Answer from the drawing. Dimensions are ordinates in mm from the lowest x, y and z of the part. Give positions to 0.01 mm unless a question says otherwise; leave off trailing zeros. Loops run counter-clockwise (first coordinate to the right, second up) from the corner with the lowest first, then second, coordinate; pieces in that order, holes last. Notation, with made-up numbers: (-17.5, 61) - (20.5, 61) arc R19 cw to (20.5, 81) - close; hole circle Ø6 at (61, 26). An arc over 180 degrees is marked (long way). Put each result on its own line as item: value. Start each with the question number.
1. A cutting plane is placed at D-D, the plane z = 47. Determine the outline of the cut face in (x, y), plus the area to 3 significant figures.
2. Consider L1, parallel to X at y = 6.5, z = 27.5; L2, parallel to Z at x = 25, y = 2.25 (1 decimal); L3, parallel to X at y = 6.75, z = 44.5 (1 decimal). Determine where each line is inside the solid, lowest interval first. Write a range as from..to.
3. A cutting plane is placed at C-C, the plane y = 2.75. Determine the outline of the cut face in (x, z) (1 decimal).
4. For a pull along Z with two mould halves and no side action, classify the marked faces 1, 2 and 3 as released by +Z, released by -Z, zero draft, split by the parting line, or undercut.
5. A cutting plane is placed at B-B, the plane x = 27.5. Determine the outline of the cut face in (y, z), plus the area to 3 significant figures.
6. Given pin 1 Ø1.5 at (y, z) = (3.5, 24) entering from -X; pin 2 Ø2 at (y, z) = (3.5, 20) entering from -X; pin 3 Ø1.2 at (x, z) = (34, 18) entering from +Y; pin 4 Ø13.5 at (x, z) = (27.5, 27.5) entering from -Y, each flat-ended and moving along its own axis, determine where each tip first touches the part or whether it passes through.
7. A cutting plane is placed at A-A, the plane z = 27.5. Determine the outline of the cut face in (x, y), plus the area to 3 significant figures.
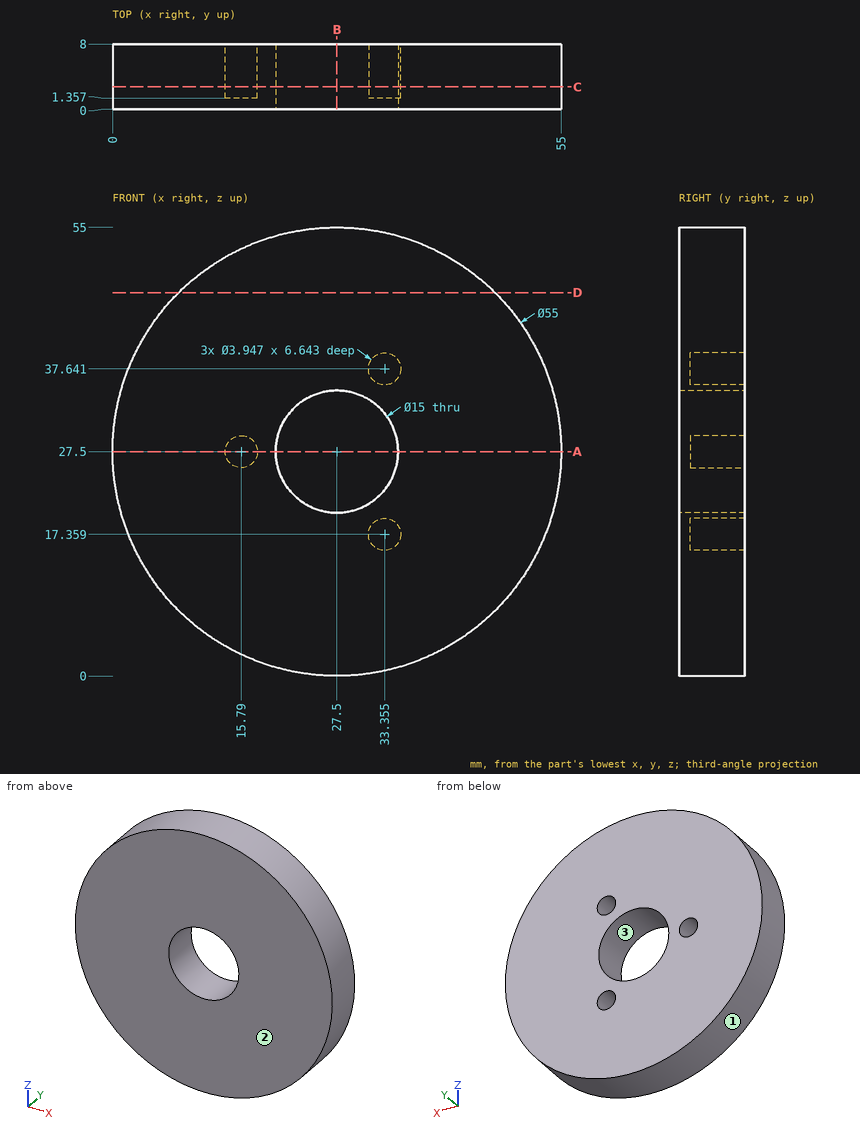
Return value:
1. outline: (8.11, 0) - (46.89, 0) - (46.89, 8) - (8.11, 8) - close
1. area: 310 mm2
2. L1: x = 0..13.82, 17.76..20, 35..55
2. L2: z = 0.1..20.4, 34.6..54.9
2. L3: x = 5.9..49.1
3. outline: circle Ø55 at (27.5, 27.5); hole circle Ø3.9 at (15.8, 27.5); hole circle Ø15 at (27.5, 27.5); hole circle Ø3.9 at (33.4, 17.4); hole circle Ø3.9 at (33.4, 37.6)
4. face 1: split by the parting line
4. face 2: zero draft
4. face 3: undercut
5. outline: (0, 0) - (8, 0) - (8, 20) - (0, 20) - close; (0, 35) - (8, 35) - (8, 55) - (0, 55) - close
5. area: 320 mm2
6. pin 1: stops at x = 0.14
6. pin 2: stops at x = 0.78
6. pin 3: stops at y = 1.36
6. pin 4: passes through
7. outline: (0, 0) - (20, 0) - (20, 8) - (17.76, 8) - (17.76, 1.36) - (13.82, 1.36) - (13.82, 8) - (0, 8) - close; (35, 0) - (55, 0) - (55, 8) - (35, 8) - close
7. area: 294 mm2
